Verification items for the finished model (mm, model axes). Round coordinates to 2 decimals unless told otherwise and drop trailing zeros. One line per item, written item: value. Start each with the question number.
Item 1: Section check A-A, the plane z = 0.75. State how many separate pieces and enclosed holes the cut face has, then the cut area to 3 significant figures.
Item 2: Thickness scan on probe 1 along Y at (x, z) = (260, -0.7); probe 2 along Y at (x, z) = (263.5, -0.3). Record the ranges inside material, lowest first. Write a range as from..to.
Item 3: Gauge pin test, flat ends, axial feed: pin 1 (1 mm diameter, centred on x = 260.5, z = 1, fed in from +Y); pin 2 (1.1 mm diameter, centred on x = 244.5, z = 1, fed in from +Y); pin 3 (0.7 mm diameter, centred on y = 0.5, z = -0.5, fed in from -X). Record the tip position at first contact, or that the pin passes through.
from build123d import *

# Parameters (mm, degrees)
SKETCH_1_W      = 5
SKETCH_1_H      = 2.8
SKETCH_1_R      = 1
EXTRUDE_1_DEPTH = 1.4


with BuildPart() as part:
    # Эскиз1 → Бобышка-Вытянуть1 (new, symmetric)
    with BuildSketch(Plane.XY):
        with BuildLine():
            ThreePointArc((223.382624747, 5.634990628), (219.398084745, 3.984540168), (217.747634119, 2.35e-07))
            ThreePointArc((217.747634119, 2.35e-07), (219.398084579, -3.984540002), (223.382624747, -5.634990628))
            add(Edge.make_bspline(
                [(223.382624747, -5.634990628), (224.328656864, -5.562010205), (226.923894547, -5.359166556), (231.150377303, -5.017351103), (236.038226964, -4.605811749), (240.854179313, -4.184912649), (247.071089236, -3.62220531), (253.116111921, -3.047869044), (258.952644662, -2.467188138), (263.047743378, -2.047856604), (266.898988862, -1.642607304), (270.455833183, -1.258590905), (273.651166984, -0.905304265), (276.385426802, -0.596436482), (278.45259621, -0.358958361), (279.592043704, -0.226075898), (280, -0.1785)],
                knots=[0.670161589, 0.670161589, 0.670161589, 0.670161589, 0.686667237, 0.715444849, 0.743923546, 0.77199483, 0.799540253, 0.852512115, 0.877624446, 0.901571134, 0.924121062, 0.944988816, 0.963803939, 0.980044339, 0.992855276, 1, 1, 1, 1], degree=3))
            ThreePointArc((280, -0.1785), (280.073937121, 0), (280, 0.1785))
            add(Edge.make_bspline(
                [(280, 0.1785), (279.592043704, 0.226075898), (278.45259621, 0.358958361), (276.385426802, 0.596436482), (273.651166984, 0.905304265), (270.455833183, 1.258590905), (266.898988862, 1.642607304), (263.047743378, 2.047856604), (258.952644662, 2.467188138), (253.116111921, 3.047869044), (247.071089236, 3.62220531), (240.854179313, 4.184912649), (236.038226964, 4.605811749), (231.150377303, 5.017351103), (226.923894547, 5.359166556), (224.328656864, 5.562010205), (223.382624747, 5.634990628)],
                knots=[0, 0, 0, 0, 0.007144724, 0.019955661, 0.036196061, 0.055011184, 0.075878938, 0.098428866, 0.122375554, 0.147487885, 0.200459747, 0.22800517, 0.256076454, 0.284555151, 0.313332763, 0.329838411, 0.329838411, 0.329838411, 0.329838411], degree=3))
        make_face()
        with Locations((243.382624747, 0)):
            Rectangle(SKETCH_1_W, SKETCH_1_H, mode=Mode.SUBTRACT)
        with Locations((223.382624747, 0)):
            Circle(SKETCH_1_R, mode=Mode.SUBTRACT)
    extrude(amount=EXTRUDE_1_DEPTH, both=True)


solid = part.part
Response values:
1. separate pieces: 1
1. enclosed holes: 2
1. area: 383 mm2
2. probe 1: y = -2.36..2.36
2. probe 2: y = -2..2
3. pin 1: stops at y = 2.36
3. pin 2: stops at y = 3.9
3. pin 3: stops at x = 217.75
